```python
from build123d import *

# Parameters (mm, degrees)
ESQUISSE1_W             = 70
ESQUISSE1_H             = 12
BOSS_EXTRU_1_DEPTH      = 80
ESQUISSE2_W             = 12
ESQUISSE2_H             = 6
ENL_V_MAT_EXTRU_1_DEPTH = 107.976632963
ESQUISSE4_R             = 2.25
ENL_V_MAT_EXTRU_3_DEPTH = 107.976632963
ESQUISSE5_W             = 12
ESQUISSE5_H             = 10
BOSS_EXTRU_2_DEPTH      = 6
CHANFREIN1_SIZE         = 3
ESQUISSE6_R             = 1
ENL_V_MAT_EXTRU_4_DEPTH = 12
ENL_V_START             = -80
ESQUISSE8_W             = 70
ESQUISSE8_H             = 9
ENL_V_MAT_EXTRU_8_DEPTH = 80


with BuildPart() as part:
    # Esquisse1 → Boss.-Extru.1 (new body)
    with BuildSketch(Plane.XY):
        with Locations((35, 6)):
            Rectangle(ESQUISSE1_W, ESQUISSE1_H)
    extrude(amount=BOSS_EXTRU_1_DEPTH)

    # Esquisse2 → Enlèv. mat.-Extru.1 (cut, through all)
    with BuildSketch(Plane.XY.offset(80)):
        with Locations((52.5, 9)):
            Rectangle(ESQUISSE2_W, ESQUISSE2_H)
        with Locations((17.5, 9)):
            Rectangle(ESQUISSE2_W, ESQUISSE2_H)
    extrude(amount=-ENL_V_MAT_EXTRU_1_DEPTH, mode=Mode.SUBTRACT)

    # Esquisse4 → Enlèv. mat.-Extru.3 (cut, through all)
    with BuildSketch(Plane(origin=(0, 12, 0), x_dir=(1, 0, 0), z_dir=(0, 1, 0))):
        with Locations(Location((5, -10, 0), (0, 0, 270))):
            Circle(ESQUISSE4_R)
        with Locations(Location((65, -70, 0), (0, 0, 270))):
            Circle(ESQUISSE4_R)
        with Locations(Location((65, -10, 0), (0, 0, 90))):
            Circle(ESQUISSE4_R)
        with Locations(Location((5, -70, 0), (0, 0, 90))):
            Circle(ESQUISSE4_R)
        with Locations(Location((35, -10, 0), (0, 0, 270))):
            Circle(ESQUISSE4_R)
        with Locations(Location((35, -70, 0), (0, 0, 270))):
            Circle(ESQUISSE4_R)
    extrude(amount=-ENL_V_MAT_EXTRU_3_DEPTH, mode=Mode.SUBTRACT)

    # Esquisse5 → Boss.-Extru.2 (add)
    with BuildSketch(Plane(origin=(0, 12, 0), x_dir=(1, 0, 0), z_dir=(0, 1, 0))):
        with Locations((17.5, -75)):
            Rectangle(ESQUISSE5_W, ESQUISSE5_H)
        with Locations((52.5, -75)):
            Rectangle(ESQUISSE5_W, ESQUISSE5_H)
        with Locations((52.5, -5)):
            Rectangle(ESQUISSE5_W, ESQUISSE5_H)
        with Locations((17.5, -5)):
            Rectangle(ESQUISSE5_W, ESQUISSE5_H)
    extrude(amount=-BOSS_EXTRU_2_DEPTH)

    # Chanfrein1
    chanfrein1_edges = [part.edges().sort_by_distance(p)[0] for p in [
        (70, 6, 80),
        (0, 6, 80),
        (70, 6, 0),
        (0, 6, 0),
    ]]
    chamfer(chanfrein1_edges, length=CHANFREIN1_SIZE)

    # Esquisse6 → Enlèv. mat.-Extru.4 (cut)
    with BuildSketch(Plane(origin=(0, 12, 0), x_dir=(1, 0, 0), z_dir=(0, 1, 0))):
        with Locations(Location((5, -20, 0), (0, 0, 270))):
            Circle(ESQUISSE6_R)
        with Locations(Location((5, -60, 0), (0, 0, 90))):
            Circle(ESQUISSE6_R)
        with Locations(Location((65, -60, 0), (0, 0, 270))):
            Circle(ESQUISSE6_R)
        with Locations(Location((65, -20, 0), (0, 0, 90))):
            Circle(ESQUISSE6_R)
    extrude(amount=-ENL_V_MAT_EXTRU_4_DEPTH, mode=Mode.SUBTRACT)

    # Esquisse8 → Enlèv. mat.-Extru.8 (cut)
    with BuildSketch(Plane.XY.offset(80).offset(ENL_V_START)):
        with Locations((35, 4.5)):
            Rectangle(ESQUISSE8_W, ESQUISSE8_H)
    extrude(amount=ENL_V_MAT_EXTRU_8_DEPTH, mode=Mode.SUBTRACT)


solid = part.part
```
Work out the finished part from the listing and answer in its coordinate system (mm). A direction names the side the tool comes from. Give positions to 0.01 mm unless a question says otherwise; leave off trailing zeros. Write each loop counter-clockwise with the first axis right and the second up, starting at its lowest first coordinate (ties: lowest second). Pieces come first, ordered by that corner, then holes.
(1) Which of the six approach directions +Z, -Z, +X, -X, +Y, -Y give full straight-line access (tool end or side, diameter ignored) to faces 4 (the flat face through (69, 10, 78)), 5 (the flat face through (46.5, 10, 40))?
Final values:
face 4: +Z, +X, +Y, -Y
face 5: +Y, -Y
(2) The part is cut by section D-D on x = 35. Write down the section's boundary in (y, z), plus the area to 3 significant figures.
Final values:
outline: (9, 0) - (12, 0) - (12, 7.75) - (9, 7.75) - close; (9, 12.25) - (12, 12.25) - (12, 67.75) - (9, 67.75) - close; (9, 72.25) - (12, 72.25) - (12, 80) - (9, 80) - close
area: 213 mm2
(3) The part is cut by section C-C on z = 60. Write down the section's boundary in (x, y), plus the area to 3 significant figures.
Final values:
outline: (0, 9) - (4, 9) - (4, 12) - (0, 12) - close; (6, 9) - (11.5, 9) - (11.5, 12) - (6, 12) - close; (23.5, 9) - (46.5, 9) - (46.5, 12) - (23.5, 12) - close; (58.5, 9) - (64, 9) - (64, 12) - (58.5, 12) - close; (66, 9) - (70, 9) - (70, 12) - (66, 12) - close
area: 126 mm2
(4) Straight lines are drawn through the part: line 1 (X direction, y = 10.7, z = 20); line 2 (X direction, y = 10, z = 44.5); line 3 (Z direction, x = 57.5, y = 11.55). For each, find the intervals that lie inside material, in ascending order.
Final values:
line 1: x = 0 to 4, 6 to 11.5, 23.5 to 46.5, 58.5 to 64, 66 to 70
line 2: x = 0 to 11.5, 23.5 to 46.5, 58.5 to 70
line 3: z = 0 to 10, 70 to 80
(5) The part is cut by section B-B on x = 65. Write down the section's boundary in (y, z).
Final values:
outline: (9, 0) - (12, 0) - (12, 7.75) - (9, 7.75) - close; (9, 12.25) - (12, 12.25) - (12, 19) - (9, 19) - close; (9, 21) - (12, 21) - (12, 59) - (9, 59) - close; (9, 61) - (12, 61) - (12, 67.75) - (9, 67.75) - close; (9, 72.25) - (12, 72.25) - (12, 80) - (9, 80) - close
(6) The mould has two halves that part along X. Classify faces 1 (the flat face through (69, 10, 2)), 2 (the cylindrical face through (5.676, 10.521, 19.263)), 3 (the flat face through (1, 10, 2)): pulls with the +X half, pulls with the -X half, needs draft (parallel to the pull), parting line crosses it, or undercut.
Final values:
face 1: pulls with the +X half
face 2: undercut
face 3: pulls with the -X half
(7) The part is cut by section A-A on z = 44.5. Write down the section's boundary in (x, y).
Final values:
outline: (0, 9) - (11.5, 9) - (11.5, 12) - (0, 12) - close; (23.5, 9) - (46.5, 9) - (46.5, 12) - (23.5, 12) - close; (58.5, 9) - (70, 9) - (70, 12) - (58.5, 12) - close
